Read the model definition and answer for the solid it produces. Units are mm, in the model's axes. Face numbers are marked on the shaded views. Coordinates: 2 decimals unless noted, no trailing zeros. Loops run counter-clockwise (first coordinate to the right, second up) from the corner with the lowest first, then second, coordinate; pieces in that order, holes last. Notation, with made-up numbers: M 88.25,12 L 130.25,12 A17 ccw 130.25,16 Z; hole C 50,61.5 d5. An arc over 180 degrees is marked long. One line per item, written item: value. Start each with the question number.
1. Determine the mould class of the marked faces 1, 2 and 3 for opening direction X: +X half, -X half, draft (parallel to the pull), parting line (faces both ways), or undercut.
2. Consider probe 1 along Y at (x, z) = (0, -7.5); probe 2 along Y at (x, z) = (0, -1.2). Determine where each line is inside the solid, lowest interval first.
3. Flat-ended cylindrical pins translate along their axes: pin 1 (6 mm diameter, centred on x = 1, z = -9, fed in from +Y); pin 2 (3 mm diameter, centred on x = 4.5, z = -10, fed in from -Y); pin 3 (1.5 mm diameter, centred on x = -4.5, z = -2.5, fed in from +Y). Find the tip coordinate at first contact, or state that the pin passes through.
4. The part is cut by section A-A (x = 0). Write down the section's boundary in (y, z), then the cut area to 3 significant figures.
5. The part is cut by section D-D (z = -4.25). Write down the section's boundary in (x, y).
6. The part is cut by section C-C (z = -6.75). Write down the section's boundary in (x, y), then the cut area to 3 significant figures.
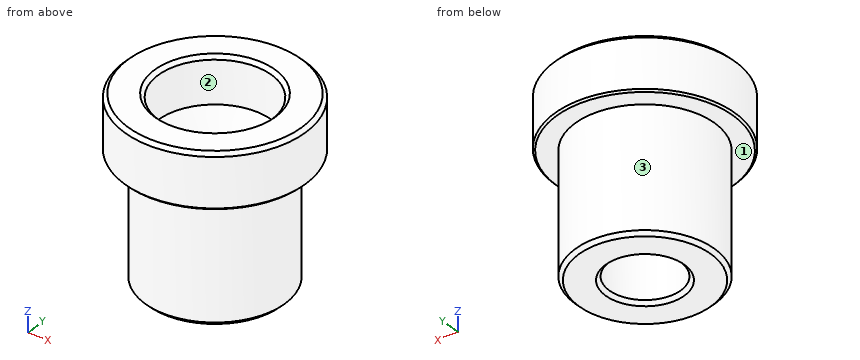
```python
from build123d import *

# Parameters (mm, degrees)
F2_SIZE     = 0.254
F3_S5_R     = 3.96875
F3_T6_DEPTH = 9
F4_SIZE     = 0.127


# Not quite as in the source:
# - a fillet or chamfer that OpenCascade refuses, or shapes differently, is made with other operations: its cross-section is extruded or revolved along the edge and cut away or added


with BuildPart() as f1:
    # F0 (on Front) → F1 (revolve)
    with BuildSketch(Plane.XZ):
        Polygon((6.3246, -3.81), (6.3246, 0), (3.96875, 0), (3.96875, -2.159), (2.50825, -2.159), (2.50825, -12.446), (4.8895, -12.446), (4.8895, -3.81), align=None)
    revolve(axis=Axis((0, 0, -10.7170343399), (0, 0, -1)))

    # F2
    f2_edges = [f1.edges().sort_by_distance(p)[0] for p in [
        (-6.3246, 0, 0),
        (-4.8895, 0, -12.446),
        (-2.50825, 0, -12.446),
        (-3.96875, 0, 0),
    ]]
    chamfer(f2_edges, length=F2_SIZE)

    # F3: chamfer of 2.54 on 1 edges, made by hand


with BuildPart() as f3_tool2:
    # F3_s3 → F3_t4 (revolve)
    with BuildSketch(Plane.XZ):
        Polygon((2.50825, -4.699), (5.04825, -2.159), (2.50825, -2.159), align=None)
    revolve(axis=Axis((0, 0, -2.159), (0, 0, -1)))

    # F3_s5 → F3_t6 (intersect, symmetric)
    with BuildSketch(Plane.XY.offset(-3.4)):
        Circle(F3_S5_R)
    extrude(amount=F3_T6_DEPTH, both=True, mode=Mode.INTERSECT)


with BuildPart() as f1_1:
    add(f1.part)

    # F3_t1: cut F3_tool2
    add(f3_tool2.part, mode=Mode.SUBTRACT)

    # F4
    f4_edges = [f1_1.edges().sort_by_distance(p)[0] for p in [
        (-6.3246, 0, -3.81),
    ]]
    chamfer(f4_edges, length=F4_SIZE)


solid = f1_1.part
```
Answer block:
1. face 1: draft
1. face 2: undercut
1. face 3: parting line
2. probe 1: y = -4.89 to -2.51, 2.51 to 4.89
2. probe 2: y = -6.32 to -3.97, 3.97 to 6.32
3. pin 1: stops at y = 4.89
3. pin 2: stops at y = -3.86
3. pin 3: stops at y = 5.09
4. outline: M -6.32,-3.68 L -6.2,-3.81 L -4.89,-3.81 L -4.89,-12.19 L -4.64,-12.45 L -2.76,-12.45 L -2.51,-12.19 L -2.51,-4.7 L -3.97,-3.24 L -3.97,-0.25 L -4.22,0 L -6.07,0 L -6.32,-0.25 Z; M 2.51,-12.19 L 2.76,-12.45 L 4.64,-12.45 L 4.89,-12.19 L 4.89,-3.81 L 6.2,-3.81 L 6.32,-3.68 L 6.32,-0.25 L 6.07,0 L 4.22,0 L 3.97,-0.25 L 3.97,-3.24 L 2.51,-4.7 Z
4. area: 58.3 mm2
5. outline: C 0,0 d9.78; hole C 0,0 d5.91
6. outline: C 0,0 d9.78; hole C 0,0 d5.02
6. area: 55.3 mm2
